Verification items for the finished model (mm, model axes). Face numbers are marked on the shaded views. A direction names the side the tool comes from. Give positions to 0.01 mm unless a question says otherwise; leave off trailing zeros. Write each loop counter-clockwise with the first axis right and the second up, starting at its lowest first coordinate (ties: lowest second). Pieces come first, ordered by that corner, then holes. Notation, with made-up numbers: (70, 40) -> (90, 40) arc R9 cw to (90, 53) -> close; hole circle Ø4 at (81, -29). An arc over 180 degrees is marked (long way). Use one line per item in the form item = value. Start each with the question number.
(1) Scan lines: L1, parallel to Y at x = 60, z = 11.25 (3 decimals); L2, parallel to Y at x = 58, z = 8.5; L3, parallel to Z at x = 5, y = 14 (3 decimals). Record each from-to range of solid material in increasing order.
(2) Section check C-C, the plane x = 29. Record the cut outline in (y, z), plus the area to 3 significant figures.
(3) Section check A-A, the plane z = 7. Record the cut outline in (x, y) (3 decimals), plus the area to 3 significant figures.
(4) Set-up check for the marked faces 1, 2 and 3: record each of +Z, -Z, +X, -X, +Y, -Y from which the full face is reachable in a straight line by a thin tool's end or side.
(5) Section check B-B, the plane y = 20. Record the cut outline in (x, z) (3 decimals).
(6) Release check for a two-part mould opening along Y. For the marked faces 4, 5 and 6 record: pulls with the +Y half, pulls with the -Y half, needs draft (parallel to the pull), parting line crosses it, or undercut.
(7) Depth check by flat-ended pin: pin 1 Ø8 at (y, z) = (46.5, 10) entering from -X; pin 2 Ø3 at (x, z) = (5, 7) entering from +Y; pin 3 Ø5 at (x, z) = (4, 10.5) entering from -Y. Enter the tip coordinate at first touch or a pass-through.
(8) Section check D-D, the plane x = 60. Record the cut outline in (y, z) (3 decimals).
from build123d import *

# Parameters (mm, degrees)
F1_DEPTH = 14
F2_R     = 19.25
F2_R_2   = 2.625
F2_W     = 10
F2_H     = 10
F3_DEPTH = 25
F4_W     = 13.615144
F4_H     = 3
F5_DEPTH = 25
F6_R     = 2.625
F7_DEPTH = 40.001


with BuildPart() as f1:
    # F0 (on Top) → F1 (new body)
    with BuildSketch(Plane.XY):
        Polygon((10, 10), (10, 0), (70, 0), (70, 50), (0, 50), (0, 10), align=None)
    extrude(amount=F1_DEPTH)

    # F2 (on face) → F3 (cut)
    with BuildSketch(Plane.XY.offset(14)):
        with Locations((29, 25)):
            Circle(F2_R)
        with Locations((60, 35)):
            Circle(F2_R_2)
        with Locations((60, 15)):
            Circle(F2_R_2)
        with Locations((5, 45)):
            Rectangle(F2_W, F2_H)
    extrude(amount=-F3_DEPTH, mode=Mode.SUBTRACT)

    # F4 (on face) → F5 (cut)
    with BuildSketch(Plane.XY.offset(14)):
        with Locations((6.807572, 25)):
            Rectangle(F4_W, F4_H)
    extrude(amount=-F5_DEPTH, mode=Mode.SUBTRACT)

    # F6 (on face) → F7 (cut, through all)
    with BuildSketch(Plane.XZ.offset(-10)):
        with Locations((5, 7)):
            Circle(F6_R)
    extrude(amount=-F7_DEPTH, mode=Mode.SUBTRACT)


solid = f1.part
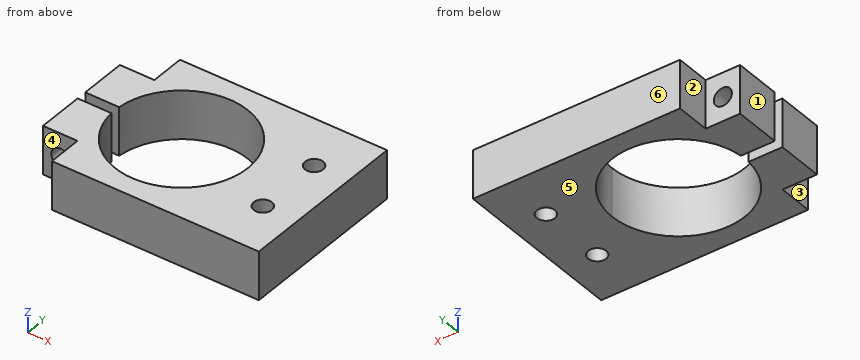
Completed:
q1.L1 = 0 to 12.375, 17.625 to 32.375, 37.625 to 50
q1.L2 = 0 to 13.3, 16.7 to 33.3, 36.7 to 50
q1.L3 = 0 to 4.375, 9.625 to 14
q2.outline = (0, 0) -> (5.75, 0) -> (5.75, 14) -> (0, 14) -> close; (44.25, 0) -> (50, 0) -> (50, 14) -> (44.25, 14) -> close
q2.area = 161 mm²
q3.outline = (0, 10) -> (2.375, 10) -> (2.375, 23.5) -> (0, 23.5) -> close; (0, 26.5) -> (2.375, 26.5) -> (2.375, 40) -> (0, 40) -> close; (7.625, 10) -> (10, 10) -> (10, 0) -> (70, 0) -> (70, 50) -> (10, 50) -> (10, 40) -> (7.625, 40) -> (7.625, 26.5) -> (9.809, 26.5) arc R19.25 cw (long way) to (9.809, 23.5) -> (7.625, 23.5) -> close; hole circle Ø5.25 at (60, 15); hole circle Ø5.25 at (60, 35)
q3.area = 1,920 mm²
q4.face_1 = +Z, -Z, -X, +Y, -Y
q4.face_2 = +Z, -Z, -X, +Y
q4.face_3 = +Z, -Z, -X, -Y
q5.outline = (0, 0) -> (10.411, 0) -> (10.411, 14) -> (0, 14) -> close; (47.589, 0) -> (70, 0) -> (70, 14) -> (47.589, 14) -> close; hole circle Ø5.25 at (5, 7)
q6.face_4 = pulls with the -Y half
q6.face_5 = needs draft
q6.face_6 = pulls with the +Y half
q7.pin_1 = 10
q7.pin_2 = through
q7.pin_3 = 10
q8.outline = (0, 0) -> (12.375, 0) -> (12.375, 14) -> (0, 14) -> close; (17.625, 0) -> (32.375, 0) -> (32.375, 14) -> (17.625, 14) -> close; (37.625, 0) -> (50, 0) -> (50, 14) -> (37.625, 14) -> close
